```python
from build123d import *

# Parameters (mm, degrees)
F0_W      = 23
F0_H      = 12
F1_DEPTH  = 26.5
F4_DEPTH  = 1.15
F5_D      = 2.4
F6_R      = 3.95
F7_DEPTH  = 3.75
F8_R      = 1.25
F9_DEPTH  = 1.8
F10_W     = 5.9
F10_H     = 3.5
F11_DEPTH = 5


with BuildPart() as f1:
    # F0 (on Top) → F1 (new body)
    with BuildSketch(Plane.XY):
        Rectangle(F0_W, F0_H)
    extrude(amount=F1_DEPTH)

    # F3 (on offset) → F4 (join)
    with BuildSketch(Plane.XY.offset(20)):
        with BuildLine():
            Line((16, 1), (16, 6))
            Line((16, 6), (-16, 6))
            Line((-16, 6), (-16, 1))
            Line((-16, 1), (-14, 1))
            ThreePointArc((-14, 1), (-13, 0), (-14, -1))
            Line((-14, -1), (-16, -1))
            Line((-16, -1), (-16, -6))
            Line((-16, -6), (16, -6))
            Line((16, -6), (16, -1))
            Line((16, -1), (14, -1))
            ThreePointArc((14, -1), (13, 0), (14, 1))
            Line((14, 1), (16, 1))
        make_face()
    extrude(amount=F4_DEPTH)

    # F5 (through all)
    with Locations(Plane(origin=(0, 0, 20), x_dir=(1, 0, 0), z_dir=(0, 0, -1))):
        with Locations((-14, 3.5), (-14, -3.5), (14, 3.5), (14, -3.5)):
            Hole(F5_D / 2)

    # F6 (on face) → F7 (join)
    with BuildSketch(Plane.XY.offset(26.5)):
        with Locations((-5.5, 0)):
            Circle(F6_R)
    extrude(amount=F7_DEPTH)

    # F8 (on face) → F9 (join)
    with BuildSketch(Plane.XY.offset(30.25)):
        with BuildLine():
            ThreePointArc((-1.56396, -0.3318), (-1.553492, -0.166047), (-1.55, 0))
            ThreePointArc((-1.55, 0), (-5.666047, 3.946508), (-9.43604, -0.3318))
            ThreePointArc((-9.43604, -0.3318), (-5.5, -3.95), (-1.56396, -0.3318))
        make_face()
        with BuildLine():
            ThreePointArc((-1.56396, -0.3318), (-5.5, -3.95), (-9.43604, -0.3318))
            Line((-9.43604, -0.3318), (-7.866606, -18.9495))
            ThreePointArc((-7.866606, -18.9495), (-5.599838, -16.377099), (-3.125, -18.75))
            ThreePointArc((-3.125, -18.75), (-3.127099, -18.849838), (-3.133394, -18.9495))
            Line((-3.133394, -18.9495), (-1.56396, -0.3318))
        make_face()
        with Locations((-5.5, -13)):
            Circle(F8_R, mode=Mode.SUBTRACT)
        with BuildLine():
            ThreePointArc((-3.125, -18.75), (-5.599838, -16.377099), (-7.866606, -18.9495))
            ThreePointArc((-7.866606, -18.9495), (-5.5, -21.125), (-3.133394, -18.9495))
            ThreePointArc((-3.133394, -18.9495), (-3.127099, -18.849838), (-3.125, -18.75))
        make_face()
    extrude(amount=F9_DEPTH)

    # F10 (on face) → F11 (join)
    with BuildSketch(Plane(origin=(-11.5, 0, 0), x_dir=(0, -1, 0), z_dir=(-1, 0, 0))):
        with Locations((0, 6.9)):
            Rectangle(F10_W, F10_H)
    extrude(amount=F11_DEPTH)


solid = f1.part
```
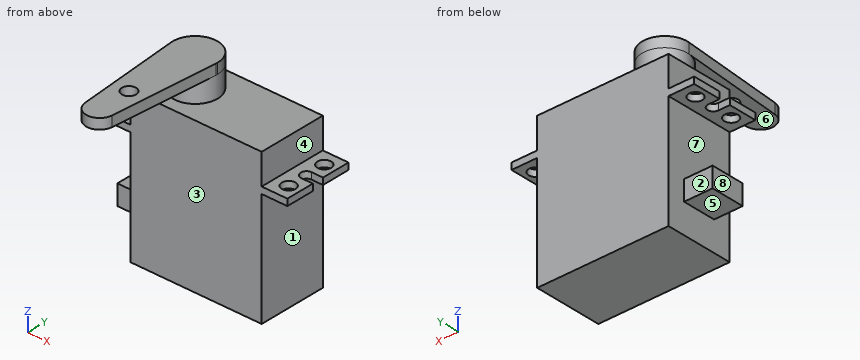
Work out the finished part from the listing and answer in its coordinate system (mm). Face numbers are marked on the shaded views. A direction names the side the tool comes from. Coordinates: 2 decimals unless noted, no trailing zeros. Loops run counter-clockwise (first coordinate to the right, second up) from the corner with the lowest first, then second, coordinate; pieces in that order, holes last.
1) Consider probe 1 along Y at (x, z) = (-14, 20.5); probe 2 along Z at (x, y) = (-7.5, -5); probe 3 along Y at (x, z) = (-6.5, 4). Determine where each line is inside the solid, lowest interval first.
Results:
probe 1: y = -6 to -4.7, -2.3 to -1, 1 to 2.3, 4.7 to 6
probe 2: z = 0 to 26.5, 30.25 to 32.05
probe 3: y = -6 to 6
2) Section B-B (y = -13) is taken. Give the vertices of the cut face in (x, z).
Results:
outline: (-8.37, 30.25) - (-6.75, 30.25) - (-6.75, 32.05) - (-8.37, 32.05) - close; (-4.25, 30.25) - (-2.63, 30.25) - (-2.63, 32.05) - (-4.25, 32.05) - close
3) Section D-D (x = 7.5) is taken. Give the vertices of the cut face in (y, z), plus the area to 3 significant figures.
Results:
outline: (-6, 0) - (6, 0) - (6, 26.5) - (-6, 26.5) - close
area: 318 mm2
4) Section C-C (z = 15) is taken. Give the vertices of the cut face in (x, y), plus the area to 3 significant figures.
Results:
outline: (-11.5, -6) - (11.5, -6) - (11.5, 6) - (-11.5, 6) - close
area: 276 mm2
5) Flat-ended cylindrical pins translate along their axes: pin 1 (1 mm diameter, centred on x = -14, z = 6, fed in from +Y); pin 2 (3 mm diameter, centred on x = -14, z = 7.5, fed in from -Y); pin 3 (4 mm diameter, centred on x = -8.5, z = 3, fed in from -Y); pin 4 (3 mm diameter, centred on y = -16, z = 28, fed in from +X). Find the tip coordinate at first contact, or state that the pin passes through.
Results:
pin 1: stops at y = 2.95
pin 2: stops at y = -2.95
pin 3: stops at y = -6
pin 4: passes through
6) Section A-A (x = -5.5) is taken. Give the vertices of the cut face in (y, z) (3 decimals), plus the area to 3 significant figures.
Results:
outline: (-21.125, 30.25) - (-14.25, 30.25) - (-14.25, 32.05) - (-21.125, 32.05) - close; (-11.75, 30.25) - (-3.95, 30.25) - (-3.95, 26.5) - (-6, 26.5) - (-6, 0) - (6, 0) - (6, 26.5) - (3.95, 26.5) - (3.95, 32.05) - (-11.75, 32.05) - close
area: 388 mm2
7) For the marked faces 1, 2, 3 and 4, determine the directions among +Z, -Z, +X, -X, +Y, -Y from which every point of the face is accessible in a straight line to the end or side of a thin tool.
Results:
face 1: -Z, +X, +Y, -Y
face 2: -Z, -X, +Y
face 3: -Z, +X, -X, -Y
face 4: +Z, +X, +Y, -Y
8) For a pull along Z with two mould halves and no side action, classify the marked faces 5, 6, 7 and 8 as +Z half, -Z half, draft (parallel to the pull), parting line (faces both ways), or undercut.
Results:
face 5: -Z half
face 6: undercut
face 7: undercut
face 8: draft
